Geometry check sheet. Reference: the model listing, model coordinates, mm. A direction names the side the tool comes from. Coordinates: 2 decimals unless noted, no trailing zeros. Loops run counter-clockwise (first coordinate to the right, second up) from the corner with the lowest first, then second, coordinate; pieces in that order, holes last.
from build123d import *

# Parameters (mm, degrees)
SKETCH_1_R          = 34
SKETCH_1_R_2        = 8
EXTRUDE_1_DEPTH     = 40.5
SKETCH_2_R          = 17.5
SKETCH_2_R_2        = 8
EXTRUDE_2_DEPTH     = 1
SKETCH_3_R          = 2.1
CUT_EXTRUDE_1_DEPTH = 5
CUT_EXTRUDE_2_DEPTH = 8
SKETCH_5_R          = 2.1
CUT_EXTRUDE_3_DEPTH = 5


with BuildPart() as part:
    # 草图1 → 凸台-拉伸1 (new body)
    with BuildSketch(Plane(origin=(0, 0, 0), x_dir=(1, 0, 0), z_dir=(0, 1, 0))):
        with Locations(Location((0, 0, 0), (0, 0, 270))):
            Circle(SKETCH_1_R)
        with Locations(Location((0, 0, 0), (0, 0, 270))):
            Circle(SKETCH_1_R_2, mode=Mode.SUBTRACT)
    extrude(amount=EXTRUDE_1_DEPTH)

    # 草图2 → 凸台-拉伸2 (add)
    with BuildSketch(Plane(origin=(0, 40.5, 0), x_dir=(1, 0, 0), z_dir=(0, 1, 0))):
        with Locations(Location((0, 0, 0), (0, 0, 270))):
            Circle(SKETCH_2_R)
        with Locations(Location((0, 0, 0), (0, 0, 270))):
            Circle(SKETCH_2_R_2, mode=Mode.SUBTRACT)
    extrude(amount=EXTRUDE_2_DEPTH)

    # 草图3 → 切除-拉伸1 (cut)
    with BuildSketch(Plane(origin=(0, 41.5, 0), x_dir=(1, 0, 0), z_dir=(0, 1, 0))):
        with Locations(Location((14, 0, 0), (0, 0, 270))):
            Circle(SKETCH_3_R)
        with Locations(Location((9.899494937, -9.899494937, 0), (0, 0, 270))):
            Circle(SKETCH_3_R)
        with Locations(Location((0, -14, 0), (0, 0, 270))):
            Circle(SKETCH_3_R)
        with Locations(Location((-9.899494937, -9.899494937, 0), (0, 0, 270))):
            Circle(SKETCH_3_R)
        with Locations(Location((-14, 0, 0), (0, 0, 270))):
            Circle(SKETCH_3_R)
        with Locations(Location((-9.899494937, 9.899494937, 0), (0, 0, 270))):
            Circle(SKETCH_3_R)
        with Locations(Location((0, 14, 0), (0, 0, 270))):
            Circle(SKETCH_3_R)
        with Locations(Location((9.899494937, 9.899494937, 0), (0, 0, 270))):
            Circle(SKETCH_3_R)
    extrude(amount=-CUT_EXTRUDE_1_DEPTH, mode=Mode.SUBTRACT)

    # 草图4 → 切除-拉伸2 (cut)
    with BuildSketch(Plane(origin=(0, 0, 0), x_dir=(-1, 0, 0), z_dir=(0, -1, 0))):
        Polygon((28.844410204, 191.136996342), (28.844410204, 18), (28.844410204, -18), (28.844410204, -191.136996342), (375.118402887, -191.136996342), (375.118402887, 191.136996342), align=None)
    extrude(amount=-CUT_EXTRUDE_2_DEPTH, mode=Mode.SUBTRACT)

    # 草图5 → 切除-拉伸3 (cut)
    with BuildSketch(Plane(origin=(0, 0, 0), x_dir=(-1, 0, 0), z_dir=(0, -1, 0))):
        with Locations(Location((-30, 0, 0), (0, 0, 90))):
            Circle(SKETCH_5_R)
        with Locations(Location((15, 25.980762114, 0), (0, 0, 90))):
            Circle(SKETCH_5_R)
        with Locations(Location((15, -25.980762114, 0), (0, 0, 90))):
            Circle(SKETCH_5_R)
    extrude(amount=-CUT_EXTRUDE_3_DEPTH, mode=Mode.SUBTRACT)


solid = part.part
1) Depth check by flat-ended pin: pin 1 (1 mm diameter, centred on y = 20, z = -17.5, fed in from -X); pin 2 (5 mm diameter, centred on x = 30, z = 0, fed in from +Y); pin 3 (2 mm diameter, centred on x = -0.5, z = 14.5, fed in from +Y); pin 4 (6.5 mm diameter, centred on x = 9.9, z = -9.9, fed in from -Y). Enter the tip coordinate at first touch or a pass-through.
Data:
pin 1: stops at x = -29.44
pin 2: stops at y = 40.5
pin 3: stops at y = 36.5
pin 4: stops at y = 0
2) Section check A-A on x = 0. Record the cut outline in (y, z).
Data:
outline: (0, -34) - (40.5, -34) - (40.5, -17.5) - (41.5, -17.5) - (41.5, -16.1) - (36.5, -16.1) - (36.5, -11.9) - (41.5, -11.9) - (41.5, -8) - (0, -8) - close; (0, 8) - (41.5, 8) - (41.5, 11.9) - (36.5, 11.9) - (36.5, 16.1) - (41.5, 16.1) - (41.5, 17.5) - (40.5, 17.5) - (40.5, 34) - (0, 34) - close
3) Section check C-C on y = 4. Record the cut outline in (x, z).
Data:
outline: (-28.84, -18) arc R34 ccw (long way) to (-28.84, 18) - close; hole circle Ø4.2 at (-15, -25.98); hole circle Ø4.2 at (-15, 25.98); hole circle Ø16 at (0, 0); hole circle Ø4.2 at (30, 0)
4) Mould release check, pull along X, two halves, no side actions. Record for faces 4 (the cylindrical face through (8, 39, 9)), 5 (the cylindrical face through (33.71, 19.97, -4.43)), 6 (the flat face through (-8, 41.5, 4)), 7 (the cylindrical face through (-14.91, 2.46, 28.08)): +X half, -X half, draft (parallel to the pull), parting line (faces both ways), or undercut.
Data:
face 4: undercut
face 5: parting line
face 6: draft
face 7: undercut
5) Access from +Z, -Z, +X, -X, +Y, -Y to the whole of each face (thin tool, end or side, straight path). Record for faces 1 (the flat face through (-15, 5, -26)), 2 (the flat face through (10, 36.5, -10)), 3 (the flat face through (3, 0, -8)).
Data:
face 1: -Y
face 2: +Y
face 3: +Z, -Z, +X, -X, -Y
6) Material ranges on probe 1 along X at (y, z) = (38.85, 0); probe 2 along X at (y, z) = (29, -0.5); probe 3 along X at (y, z) = (32, -3), recorded low to high.
Data:
probe 1: x = -34 to -16.1, -11.9 to -8, 8 to 11.9, 16.1 to 34
probe 2: x = -34 to -7.98, 7.98 to 34
probe 3: x = -33.87 to -7.42, 7.42 to 33.87
7) Section check B-B on z = 0. Record the cut outline in (x, y), and give its area (3 significant figures).
Data:
outline: (-34, 8) - (-28.84, 8) - (-28.84, 0) - (-8, 0) - (-8, 41.5) - (-11.9, 41.5) - (-11.9, 36.5) - (-16.1, 36.5) - (-16.1, 41.5) - (-17.5, 41.5) - (-17.5, 40.5) - (-34, 40.5) - close; (8, 0) - (27.9, 0) - (27.9, 5) - (32.1, 5) - (32.1, 0) - (34, 0) - (34, 40.5) - (17.5, 40.5) - (17.5, 41.5) - (16.1, 41.5) - (16.1, 36.5) - (11.9, 36.5) - (11.9, 41.5) - (8, 41.5) - close
area: 2,020 mm2
8) Section check D-D on x = -14. Record the cut outline in (y, z).
Data:
outline: (0, -30.98) - (40.5, -30.98) - (40.5, -10.5) - (41.5, -10.5) - (41.5, -2.1) - (36.5, -2.1) - (36.5, 2.1) - (41.5, 2.1) - (41.5, 10.5) - (40.5, 10.5) - (40.5, 30.98) - (0, 30.98) - (0, 27.83) - (5, 27.83) - (5, 24.13) - (0, 24.13) - (0, -24.13) - (5, -24.13) - (5, -27.83) - (0, -27.83) - close
